Verification items for the finished model (mm, model axes). Face numbers are marked on the shaded views. A direction names the side the tool comes from. Round coordinates to 2 decimals unless told otherwise and drop trailing zeros. Order: outer loops, then holes, each group sorted by start corner. A loop starts at its lowest first (then second) coordinate and runs counter-clockwise, first axis right, second up. Notation, with made-up numbers: (36, -13) -> (49, -13) arc R13 ccw to (49, -5) -> close; hole circle Ø2 at (-10, -27). An arc over 180 degrees is marked (long way). Put each result on its own line as item: value.
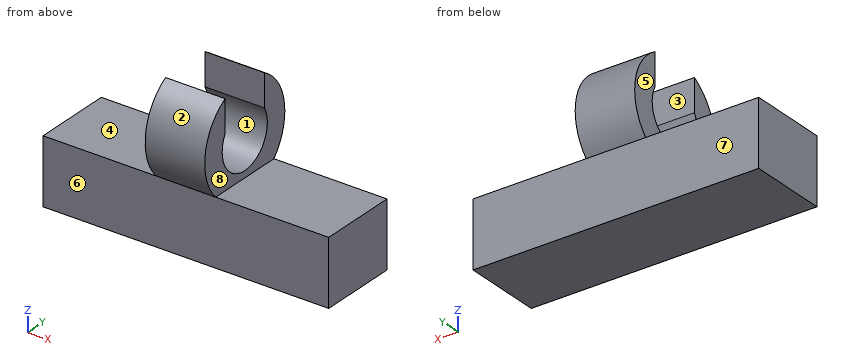
from build123d import *

# Parameters (mm, degrees)
F0_W     = 18.288
F0_H     = 5.08
F0_W_2   = 16.256
F0_H_2   = 3.302
F1_DEPTH = 3.175
F2_W     = 16.256
F2_H     = 3.302
F3_DEPTH = 0.508
F4_W     = 18.288
F4_H     = 5.08
F4_W_2   = 16.256
F4_H_2   = 3.302
F5_DEPTH = 1.016
F7_DEPTH = 1.905


with BuildPart() as f1:
    # F0 (on Top) → F1 (new body)
    with BuildSketch(Plane.XY):
        with Locations((0, 2.54)):
            Rectangle(F0_W, F0_H)
        with Locations((0, 2.54)):
            Rectangle(F0_W_2, F0_H_2, mode=Mode.SUBTRACT)
    extrude(amount=F1_DEPTH)

    # F2 (on face) → F3 (join)
    with BuildSketch(Plane(origin=(0, 0, 0), x_dir=(1, 0, 0), z_dir=(0, 0, -1))):
        with Locations((0, -2.54)):
            Rectangle(F2_W, F2_H)
    extrude(amount=-F3_DEPTH)

    # F4 (on face) → F5 (join)
    with BuildSketch(Plane.XY.offset(3.175)):
        with Locations((0, 2.54)):
            Rectangle(F4_W, F4_H)
        with Locations((0, 2.54)):
            Rectangle(F4_W_2, F4_H_2, mode=Mode.SUBTRACT)
        with Locations((0, 2.54)):
            Rectangle(F4_W_2, F4_H_2)
    extrude(amount=F5_DEPTH)

    # F6 (on Right) → F7 (join, symmetric)
    with BuildSketch(Plane.YZ):
        with BuildLine():
            Line((0, 4.191), (5.08, 4.191))
            ThreePointArc((5.08, 4.191), (5.7856514177, 5.2983813365), (6.0325, 6.5880724332))
            ThreePointArc((6.0325, 6.5880724332), (5.5554143579, 8.3501259227), (4.2545, 9.6307761651))
            Line((4.2545, 9.6307761651), (4.2545, 7.5552756176))
            ThreePointArc((4.2545, 7.5552756176), (4.4439413725, 7.0880719332), (4.5085, 6.5880724332))
            ThreePointArc((4.5085, 6.5880724332), (2.0400005, 4.6841310607), (0.8255, 7.5552756176))
            Line((0.8255, 7.5552756176), (0.8255, 9.6307761651))
            ThreePointArc((0.8255, 9.6307761651), (-0.9129673824, 7.1120690992), (0, 4.191))
        make_face()
    extrude(amount=F7_DEPTH, both=True)


solid = f1.part
Item 1: Section check C-C on y = 2.54. Record the boundary of the cut face in (x, z) (3 decimals).
Check sheet entries:
outline: (-9.144, 0) -> (9.144, 0) -> (9.144, 4.191) -> (1.905, 4.191) -> (1.905, 4.62) -> (-1.905, 4.62) -> (-1.905, 4.191) -> (-9.144, 4.191) -> close; hole (-8.128, 0.508) -> (8.128, 0.508) -> (8.128, 3.175) -> (-8.128, 3.175) -> close
Item 2: Tool access check on the marked faces 5, 6, 7 and 8. Record the directions out of +Z, -Z, +X, -X, +Y, -Y that give a thin tool (end or side, any length) a straight path to the whole face; none if there is none.
Check sheet entries:
face 5: +Z, -X, +Y, -Y
face 6: -Z, +X, -X, -Y
face 7: -Z, +X, -X, +Y
face 8: +Z, +X, +Y, -Y
Item 3: Material ranges on L1, parallel to Z at x = -4.5, y = 2.5 (3 decimals); L2, parallel to Y at x = 5.75, z = 1.25; L3, parallel to Z at x = -0.15, y = 2.54 (3 decimals), recorded low to high. Write a range as [from, to].
Check sheet entries:
L1: z = [0, 0.508], [3.175, 4.191]
L2: y = [0, 0.89], [4.19, 5.08]
L3: z = [0, 0.508], [3.175, 4.62]
Item 4: Gauge pin test, flat ends, axial feed: pin 1 Ø1.7 at (x, y) = (1.5, 3) entering from +Z; pin 2 Ø1.3 at (x, z) = (1.5, 1) entering from -Y; pin 3 Ø3.5 at (x, z) = (-1, 1.5) entering from +Y. Record the tip position at first contact, or that the pin passes through.
Check sheet entries:
pin 1: stops at z = 5.12
pin 2: stops at y = 0
pin 3: stops at y = 5.08
Item 5: Release check for a two-part mould opening along Y. For the marked faces 1, 2, 3 and 4 record: +Y half, -Y half, draft (parallel to the pull), parting line (faces both ways), or undercut.
Check sheet entries:
face 1: undercut
face 2: -Y half
face 3: undercut
face 4: draft
Item 6: Section check A-A on x = 6. Record the boundary of the cut face in (y, z) (3 decimals).
Check sheet entries:
outline: (0, 0) -> (5.08, 0) -> (5.08, 4.191) -> (0, 4.191) -> close; hole (0.889, 0.508) -> (4.191, 0.508) -> (4.191, 3.175) -> (0.889, 3.175) -> close
Item 7: Section check D-D on z = 9.25. Record the boundary of the cut face in (x, y) (1 decimal), then the cut area to 3 significant figures.
Check sheet entries:
outline: (-1.9, 0.3) -> (1.9, 0.3) -> (1.9, 0.8) -> (-1.9, 0.8) -> close; (-1.9, 4.3) -> (1.9, 4.3) -> (1.9, 4.8) -> (-1.9, 4.8) -> close
area: 4.16 mm^2
Item 8: Section check B-B on z = 3. Record the boundary of the cut face in (x, y).
Check sheet entries:
outline: (-9.14, 0) -> (9.14, 0) -> (9.14, 5.08) -> (-9.14, 5.08) -> close; hole (-8.13, 0.89) -> (8.13, 0.89) -> (8.13, 4.19) -> (-8.13, 4.19) -> close
